Geometry check sheet. Reference: the model listing, model coordinates, mm. A direction names the side the tool comes from. Give positions to 0.01 mm unless a question says otherwise; leave off trailing zeros. Write each loop counter-clockwise with the first axis right and the second up, starting at its lowest first coordinate (ties: lowest second). Pieces come first, ordered by that corner, then holes. Notation, with made-up numbers: M 27.5,76.5 L 75.5,76.5 A13 ccw 75.5,83.5 Z; hole C -13,80 d6. An arc over 180 degrees is marked long. Write each question's results on one line, items separated by ' | '.
```python
from build123d import *

# Parameters (mm, degrees)
F1_DEPTH = 13
F2_R     = 4.25
F2_R_2   = 2.5
F3_DEPTH = 14
F5_W     = 30.750612
F5_H     = 1.5
F6_DEPTH = 7.5


with BuildPart() as f1:
    # F0 (on Front) → F1 (new body, symmetric)
    with BuildSketch(Plane.XZ):
        Polygon((-15.375306, -11.020302), (-15.375306, -8.878698), (-15.375306, 8.878698), (-15.375306, 10.979698), (-24.375306, 10.979698), (-27.375306, 2.979698), (-58.375306, 2.979698), (-58.375306, -3.020302), (-27.375306, -3.020302), (-24.375306, -11.020302), align=None)
    extrude(amount=F1_DEPTH, both=True)

    # F2 (on face) → F3 (cut, through all)
    with BuildSketch(Plane.XY.offset(2.979698)):
        with Locations((-42.5, 0)):
            Circle(F2_R)
        with Locations((-19.875306, 0)):
            Circle(F2_R_2)
    extrude(amount=-F3_DEPTH, mode=Mode.SUBTRACT)



with BuildPart() as f4_1:
    # F4: instance of F1
    add(f1.part.mirror(Plane.YZ))


with BuildPart() as f1_1:
    add(f1.part)

    add(f4_1.part)  # F6 merges F4_1
    # F5 (on Top) → F6 (join, symmetric)
    with BuildSketch(Plane.XY):
        with Locations((0, 9.75)):
            Rectangle(F5_W, F5_H)
        with Locations((0, -9.75)):
            Rectangle(F5_W, F5_H)
    extrude(amount=F6_DEPTH, both=True)


solid = f1_1.part
```
Q1. Section check D-D (y = 0). State how many separate pieces and enclosed holes the cut face has, then the cut area to 3 significant figures.
Answer key:
separate pieces: 4 | enclosed holes: 0 | area: 610 mm2
Q2. Access from +Z, -Z, +X, -X, +Y, -Y to the whole of each face (thin tool, end or side, straight path). Record for faces 4 (the face through (17.49, 0.75, -3.92)), 5 (the face through (0, 10.5, 0)), 6 (the face through (0, -9, 0)), 7 (the face through (0, -10.5, 0)).
Answer key:
face 4: -Z | face 5: +Z, -Z, +Y | face 6: +Z, -Z | face 7: +Z, -Z, -Y
Q3. Section check A-A (y = -7.75). Enter the section's corners in (x, z).
Answer key:
outline: M -58.38,-3.02 L -27.38,-3.02 L -24.38,-11.02 L -15.38,-11.02 L -15.38,10.98 L -24.38,10.98 L -27.38,2.98 L -58.38,2.98 Z; M 15.38,-11.02 L 24.38,-11.02 L 27.38,-3.02 L 58.38,-3.02 L 58.38,2.98 L 27.38,2.98 L 24.38,10.98 L 15.38,10.98 Z
Q4. Material ranges on probe 1 along Y at (x, z) = (-20, 1.5); probe 2 along Y at (x, z) = (42.5, 1.15); probe 3 along X at (y, z) = (4.75, -1.25), recorded low to high. Write a range as [from, to].
Answer key:
probe 1: y = [-13, -2.5], [2.5, 13] | probe 2: y = [-13, -4.25], [4.25, 13] | probe 3: x = [-58.38, -15.38], [15.38, 58.38]
Q5. Section check B-B (x = -42.5). Enter the section's corners in (y, z), then the cut area to 3 significant figures.
Answer key:
outline: M -13,-3.02 L -4.25,-3.02 L -4.25,2.98 L -13,2.98 Z; M 4.25,-3.02 L 13,-3.02 L 13,2.98 L 4.25,2.98 Z | area: 105 mm2
Q6. Section check C-C (z = 0). Enter the section's corners in (x, y), then the cut area to 3 significant figures.
Answer key:
outline: M -58.38,-13 L -15.38,-13 L -15.38,-10.5 L 15.38,-10.5 L 15.38,-13 L 58.38,-13 L 58.38,13 L 15.38,13 L 15.38,10.5 L -15.38,10.5 L -15.38,13 L -58.38,13 Z; hole C -42.5,0 d8.5; hole C -19.88,0 d5; hole M -15.38,-9 L 15.38,-9 L 15.38,9 L -15.38,9 Z; hole C 19.88,0 d5; hole C 42.5,0 d8.5 | area: 2,180 mm2
Q7. Release check for a two-part mould opening along X. For faces 1 (the face through (0, 9, 0)), 2 (the face through (-25.9, -0.18, -6.96)), 3 (the face through (32, 13, 0)) record: released by +X, released by -X, zero draft, split by the parting line, or undercut.
Answer key:
face 1: undercut | face 2: released by -X | face 3: zero draft
Q8. Depth check by flat-ended pin: P1, Ø3, axis at x = -4.5, y = 10.5, coming from the -Z side; P2, Ø4, axis at x = -32.5, y = -6.5, coming from the -Z side; P3, Ø1.5, axis at x = 19, y = 0.5, coming from the -Z side. Enter the tip coordinate at first touch or a pass-through.
Answer key:
P1: stops at z = -7.5 | P2: stops at z = -3.02 | P3: stops at z = 2.98
